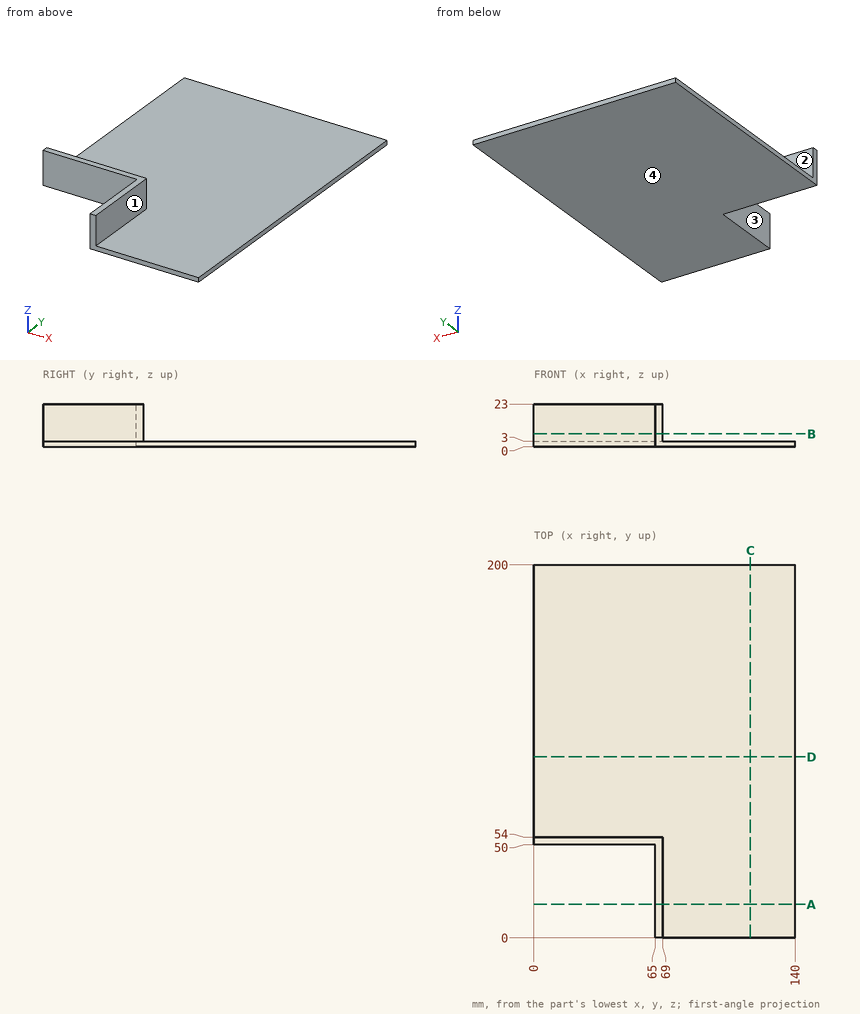
Geometry check sheet. Reference: drawing and pictorial views, mm from the part's lowest x, y, z. A direction names the side the tool comes from. Give positions to 0.01 mm unless a question says otherwise; leave off trailing zeros. Order: outer loops, then holes, each group sorted by start corner. A loop starts at its lowest first (then second) coordinate and runs counter-clockwise, first axis right, second up. Notation, with made-up numbers: (67.25, 89) -> (78.25, 89) arc R10 cw to (78.25, 98) -> close; hole circle Ø8 at (16.25, 68.25). An arc over 180 degrees is marked (long way). Use CSV: the item, a comma, the result in double quotes. Start each with the question number.
1) Sectioned sample at D-D, the plane y = 97. Record the boundary of the cut face in (x, z), plus the area to 3 significant figures.
2) Sectioned sample at B-B, the plane z = 7. Record the boundary of the cut face in (x, y).
3) Set-up check for the marked faces 1, 2, 3 and 4: record each of +Z, -Z, +X, -X, +Y, -Y from which the full face is reachable in a straight line by a thin tool's end or side.
4) Sectioned sample at A-A, the plane y = 18. Record the boundary of the cut face in (x, z), plus the area to 3 significant figures.
5) Go/stop test with flat-tipped pins: P1, Ø6, axis at x = 18.5, y = 148, coming from the +Z side; P2, Ø4, axis at y = 105.5, z = 6, coming from the +X side; P3, Ø3, axis at y = 42, z = 20.5, coming from the +X side; P4, Ø7, axis at x = 24.5, z = 11.5, coming from the -Y side. Record where each tip stops, or that it passes through.
6) Material ranges on line 1 (Z direction, x = 57.5, y = 155.5); line 2 (Y direction, x = 7, z = 3.25), recorded low to high. Write a range as from..to.
7) Sectioned sample at C-C, the plane x = 116. Record the boundary of the cut face in (y, z), plus the area to 3 significant figures.
Recorded:
1,outline,"(0, 0) -> (140, 0) -> (140, 3) -> (0, 3) -> close"
1,area,"420 mm2"
2,outline,"(0, 50) -> (65, 50) -> (65, 0) -> (69, 0) -> (69, 54) -> (0, 54) -> close"
3,face 1,"+Z, +X, +Y, -Y"
3,face 2,"+Z, +X, -X, +Y"
3,face 3,"+Z, -Z, -X, -Y"
3,face 4,"-Z, +X, -X, +Y, -Y"
4,outline,"(65, 0) -> (140, 0) -> (140, 3) -> (69, 3) -> (69, 23) -> (65, 23) -> close"
4,area,"305 mm2"
5,P1,"z = 3"
5,P2,"through"
5,P3,"x = 69"
5,P4,"y = 50"
6,line 1,"0..3"
6,line 2,"50..54"
7,outline,"(0, 0) -> (200, 0) -> (200, 3) -> (0, 3) -> close"
7,area,"600 mm2"
